Could you check a few things on this model? Use its own coordinates, in mm. Face numbers are marked on the shaded views. Give positions to 0.01 mm unless a question says otherwise; leave off trailing zeros. Order: outer loops, then holes, each group sorted by start corner. A loop starts at its lowest first (then second) coordinate and runs counter-clockwise, first axis right, second up.
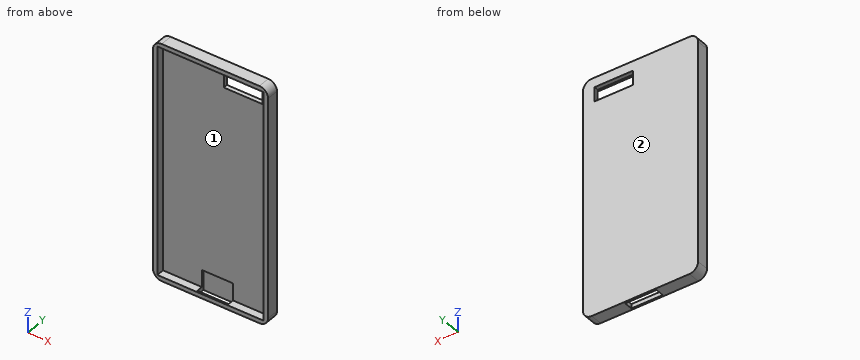
from build123d import *

# Parameters (mm, degrees)
F0_W     = 67.1
F0_H     = 138.3
F1_DEPTH = 7.1
F2_T     = -2.54
F3_R     = 5.08
F5_W     = 18.216582
F5_H     = 4.952895
F6_DEPTH = 12.5
F4_W     = 22.377047
F4_H     = 8.319672
F7_DEPTH = 12.5


with BuildPart() as f1:
    # F0 (on Front) → F1 (new body)
    with BuildSketch(Plane.XZ):
        Rectangle(F0_W, F0_H)
    extrude(amount=F1_DEPTH)

    # F2
    f2_openings = [f1.faces().sort_by_distance(p)[0] for p in [
        (0, -7.1, 0),
    ]]
    offset(amount=F2_T, openings=f2_openings)

    # F3
    f3_edges = [f1.edges().sort_by_distance(p)[0] for p in [
        (33.55, -3.55, 69.15),
        (33.55, -3.55, -69.15),
        (-33.55, -3.55, 69.15),
        (-33.55, -3.55, -69.15),
    ]]
    fillet(f3_edges, radius=F3_R)

    # F5 (on face) → F6 (cut, symmetric)
    with BuildSketch(Plane(origin=(0, 0, -69.15), x_dir=(1, 0, 0), z_dir=(0, 0, -1))):
        with Locations((0.68537, 3.650227)):
            Rectangle(F5_W, F5_H)
    extrude(amount=F6_DEPTH, both=True, mode=Mode.SUBTRACT)

    # F4 (on face) → F7 (cut, symmetric)
    with BuildSketch(Plane.XZ.offset(2.54)):
        with Locations((15.635246, 59.385249)):
            Rectangle(F4_W, F4_H)
    extrude(amount=F7_DEPTH, both=True, mode=Mode.SUBTRACT)


solid = f1.part
Item 1: Imagine slicing it at B-B on z = -7. List the corners of the cut face in (x, y) for me.
Findings:
outline: (-33.55, -7.1) - (-31.01, -7.1) - (-31.01, -2.54) - (31.01, -2.54) - (31.01, -7.1) - (33.55, -7.1) - (33.55, 0) - (-33.55, 0) - close
Item 2: Imagine slicing it at D-D on y = -4.75. List the corners of the cut face in (x, z) for me, then the cut area to 3 significant figures.
Findings:
outline: (-33.55, -64.07) arc R5.08 ccw to (-28.47, -69.15) - (-8.42, -69.15) - (-8.42, -66.61) - (-31.01, -66.61) - (-31.01, 66.61) - (31.01, 66.61) - (31.01, -66.61) - (9.79, -66.61) - (9.79, -69.15) - (28.47, -69.15) arc R5.08 ccw to (33.55, -64.07) - (33.55, 64.07) arc R5.08 ccw to (28.47, 69.15) - (-28.47, 69.15) arc R5.08 ccw to (-33.55, 64.07) - close
area: 949 mm2
Item 3: We'd pull the mould along X, two halves only. Please class the marked faces 1 and 2: +X half, -X half, draft (parallel to the pull), parting line (faces both ways), or undercut.
Findings:
face 1: undercut
face 2: draft
Item 4: Imagine slicing it at A-A on x = 13. List the corners of the cut face in (y, z) for me.
Findings:
outline: (-7.1, -69.15) - (0, -69.15) - (0, 55.23) - (-2.54, 55.23) - (-2.54, -66.61) - (-7.1, -66.61) - close; (-7.1, 66.61) - (-2.54, 66.61) - (-2.54, 63.55) - (0, 63.55) - (0, 69.15) - (-7.1, 69.15) - close
Item 5: For pin 1 (1 mm diameter, centred on x = 5, y = -2.5, fed in from -Z); pin 2 (14 mm diameter, centred on x = -1.5, z = -62.5, fed in from -Y); pin 3 (8 mm diameter, centred on x = -25, z = 24.5, fed in from -Y); pin 4 (2 mm diameter, centred on x = 7.5, y = -4, fed in from -Z), each with a flat end and sliding along its axis, tell me the tip position at first contact or that it passes through.
Findings:
pin 1: stops at z = -56.65
pin 2: stops at y = -7.1
pin 3: stops at y = -2.54
pin 4: stops at z = 66.61
Item 6: Please list where these lines run through material, in increasing order: line 1 along X through (y, z) = (-5, -33); line 2 along Z through (x, y) = (-13, -3.75).
Findings:
line 1: x = -33.55 to -31.01, 31.01 to 33.55
line 2: z = -69.15 to -66.61, 66.61 to 69.15
Item 7: Imagine slicing it at C-C on x = 1. List the corners of the cut face in (y, z) for me, then the cut area to 3 significant figures.
Findings:
outline: (-7.1, -69.15) - (-6.13, -69.15) - (-6.13, -66.61) - (-7.1, -66.61) - close; (-7.1, 66.61) - (-2.54, 66.61) - (-2.54, -56.65) - (-1.17, -56.65) - (-1.17, -69.15) - (0, -69.15) - (0, 69.15) - (-7.1, 69.15) - close
area: 348 mm2
